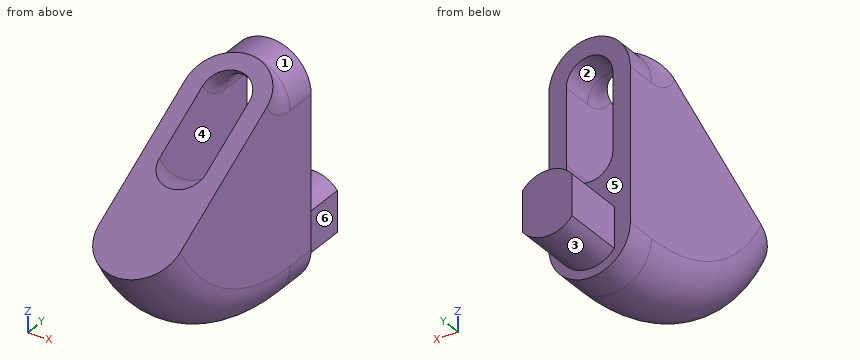
Autodesk Inventor part; units mm, degrees
ref_plane "YZ Plane" through (0, 0, 0) normal (1, 0, 0) x (0, 1, 0)
ref_plane "XZ Plane" through (0, 0, 0) normal (0, 1, 0) x (-1, 0, 0)
ref_plane "XY Plane" through (0, 0, 0) normal (0, 0, 1) x (1, 0, 0)
sketch "Schizzo1" plane through (0, 0, 0) normal (0, 1, 0) x (-1, 0, 0)
  line L0 (0, 0) -> (0, -52)
  arc A0 (0, -52) -> (28, -52) centre (14, -52) ccw
  line L1 (28, -52) -> (28, 0)
  arc A1 (28, 0) -> (0, 0) centre (14, 0) ccw
  line L2 (22, 0) -> (22, -26)
  arc A2 (22, 0) -> (6, 0) centre (14, 0) ccw
  line L3 (6, 0) -> (6, -26)
  arc A3 (6, -26) -> (22, -26) centre (14, -26) ccw
  circle A4 centre (14, -52) radius 11
  line L4 (22.5, -45.0179) -> (22.5, -58.9821)
  line L5 (5.5, -45.0179) -> (5.5, -58.9821)
  dimension "d0" = 22
  dimension "d3" = 8.5
  dimension "d4" = 8.5
  dimension "d5" = 28
  dimension "d6" = 16
  dimension "d7" = 26
  dimension "d8" = 52
extrude "Estrusione1" add sketch "Schizzo1" along normal blind 33 contours L4 A4 L5
extrude "Estrusione2" add sketch "Schizzo1" along normal blind 11 contours A1 L1 A0 L0 | A4 L4 | L5 A4
sketch "Schizzo4" plane through (0, 0, 0) normal (0, -1, 0) x (1, 0, 0)
  arc A0 (0, 0) -> (-28, 0) centre (-14, 0) ccw
  line L0 (-28, 0) -> (-28, -51.655)
  arc A1 (-28, -52) -> (0, -52) centre (-14, -52) ccw
  line L1 (-28, -51.655) -> (-28, -52)
  arc A2 (-28, -52) -> (0, -52) centre (-14, -52) ccw
  line L2 (0, 0) -> (0, -52)
  line L3 (0, -52) -> (0, 0)
  arc A3 (0, 0) -> (-28, 0) centre (-14, 0) ccw
  line L4 (0, 14) -> (-28, 14)
  arc A4 (-22, -26) -> (-6, -26) centre (-14, -26) ccw
  line L5 (-22, -26) -> (-22, 0)
  arc A5 (-22, -26) -> (-6, -26) centre (-14, -26) ccw
  line L6 (-6, -26) -> (-6, 0)
  line L7 (-6, -26) -> (-6, 0)
  arc A6 (-6, 0) -> (-22, 0) centre (-14, 0) ccw
revolve "Rivoluzione1" add sketch "Schizzo4" angle 60 about axis through (0, 0, 14) along (-1, 0, 0)
properties part number "esercizio2 02-27-2023"
Model file for the job. Use its own axes, mm. Face numbers are marked on the shaded views. A direction names the side the tool comes from. Coordinates: 2 decimals unless noted, no trailing zeros. Order: outer loops, then holes, each group sorted by start corner. A loop starts at its lowest first (then second) coordinate and runs counter-clockwise, first axis right, second up. Notation, with made-up numbers: M -9.5,-28.5 L 26.5,-28.5 A19 ccw 26.5,-9.5 Z; hole C 31.25,27 d8. An arc over 180 degrees is marked long. Answer as CSV lines item,"result".
(1) Band-saw the part on A-A, the plane y = 13. List the corners of the cut face in (x, z).
Geometry says:
outline,"M -22.5,-58.98 A11 ccw -5.5,-58.98 L -5.5,-45.02 A11 ccw -22.5,-45.02 Z"
(2) Wall check: line 1 along X through (y, z) = (-6, -13); line 2 along X through (y, z) = (21.5, -45); line 3 along X through (y, z) = (5, 6). Give the ranges that are in metal, low to high.
Geometry says:
line 1,"x = -28 to -22, -6 to 0"
line 2,"x = -22.49 to -5.51"
line 3,"x = -26.65 to -19.29, -8.71 to -1.35"
(3) Flat gauge pins, fed straight in: pin 1 (2 mm diameter, centred on y = -32, z = -25.5, fed in from +X); pin 2 (15.5 mm diameter, centred on y = 20, z = -53.5, fed in from +X); pin 3 (1.5 mm diameter, centred on x = -17, y = -3.5, fed in from +Z); pin 4 (4 mm diameter, centred on x = -13.5, z = -13.5, fed in from -Y). Where does each tip first touch, or does it go through?
Geometry says:
pin 1,"stops at x = 0"
pin 2,"stops at x = -5.5"
pin 3,"stops at z = 12.41"
pin 4,"stops at y = -51.1"
(4) Pull direction X, two halves, no side cores. Call the marked faces 4, 5 and 6: +X half, -X half, draft (parallel to the pull), parting line (faces both ways), or undercut.
Geometry says:
face 4,"undercut"
face 5,"draft"
face 6,"+X half"
(5) 3-axis set-ups, long thin cutter, end or side, ignore diameter. For the marked faces 1, 2 and 3: which of +Z, -Z, +X, -X, +Y, -Y reach the whole face in a straight line?
Geometry says:
face 1,"+Z, +Y"
face 2,"+Y, -Y"
face 3,"-Z, +Y"
